Autodesk Inventor part; units mm, degrees
ref_plane "YZ Plane" through (0, 0, 0) normal (1, 0, 0) x (0, 1, 0)
ref_plane "XZ Plane" through (0, 0, 0) normal (0, 1, 0) x (-1, 0, 0)
ref_plane "XY Plane" through (0, 0, 0) normal (0, 0, 1) x (1, 0, 0)
sketch "Sketch1" plane through (0, 0, 0) normal (1, 0, 0) x (0, 1, 0)
  line L0 (0, 0) -> (500, 0)
  line L1 (500, 0) -> (500, 270)
  line L2 (500, 270) -> (0, 270)
  line L3 (0, 270) -> (0, 0)
  dimension "d0" = 500
  dimension "d1" = 270
extrude "Extrusion1" add sketch "Sketch1" along normal blind 500
shell "Shell1" thickness 2 removed faces 1 at (333.3333, 333.3333, 270)
sketch "Sketch2" plane through (0, 500, 270) normal (0, 1, 0) x (1, 0, 0)
  point P0 (0, 270)
sketch "Sketch3" plane through (2, 498, 2) normal (0, -1, 0) x (1, 0, 0)
  line L0 (0, 268) -> (496, 268)
  line L1 (496, 0) -> (496, 268)
  line L2 (0, 268) -> (496, 268)
  line L3 (496, 268) -> (496, 266)
  line L4 (496, 266) -> (0, 266)
  line L5 (0, 266) -> (0, 268)
  point P0 (-2, -2)
  dimension "d5" = 2
extrude "Extrusion2" add sketch "Sketch3" along normal blind 496
properties part number "Caja grande"
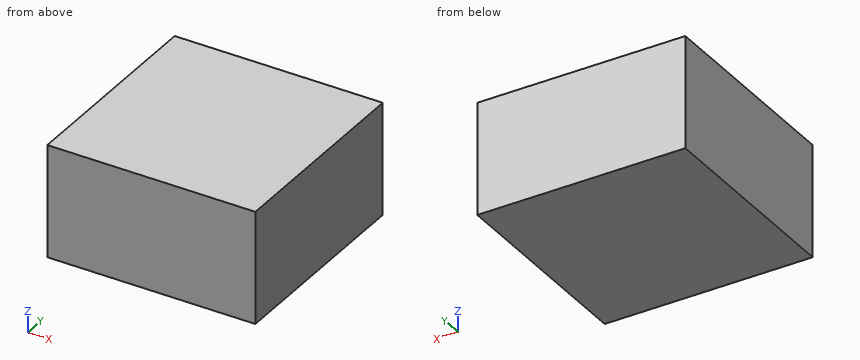
Verification items for the finished model (mm, model axes). Coordinates: 2 decimals unless noted, no trailing zeros. Order: outer loops, then holes, each group sorted by start corner. A loop starts at its lowest first (then second) coordinate and runs counter-clockwise, first axis right, second up. Notation, with made-up numbers: (54.5, -1) -> (62.5, -1) arc R11 ccw to (62.5, 16) -> close; hole circle Ø2 at (37, 56.25). An arc over 180 degrees is marked (long way). Put each result on its own line as item: value. Start each with the question number.
1. Material ranges on L1, parallel to X at y = 108, z = 113.5; L2, parallel to Z at x = 125, y = 178, recorded low to high. Write a range as [from, to].
2. Cross-section at A-A, the plane y = 127.5. Record the boundary of the cut face in (x, z), then the cut area to 3 significant figures.
Computed:
1. L1: [0, 2], [498, 500]
1. L2: [0, 2], [268, 270]
2. outline: (0, 0) -> (500, 0) -> (500, 270) -> (0, 270) -> close; hole (2, 2) -> (498, 2) -> (498, 268) -> (2, 268) -> close
2. area: 3,060 mm2
